CAD build for the part. Positions are in the model's coordinates, mm. Round coordinates to 2 decimals unless told otherwise and drop trailing zeros. Write each loop counter-clockwise with the first axis right and the second up, starting at its lowest first coordinate (ties: lowest second). Pieces come first, ordered by that corner, then holes. Notation, with made-up numbers: (57.5, 21) -> (74.5, 21) arc R34 ccw to (74.5, 56) -> close; hole circle Ø2 at (-29, 36.25). An arc over 180 degrees is marked (long way). Answer in a Markdown table with one row per item. Add a question column.
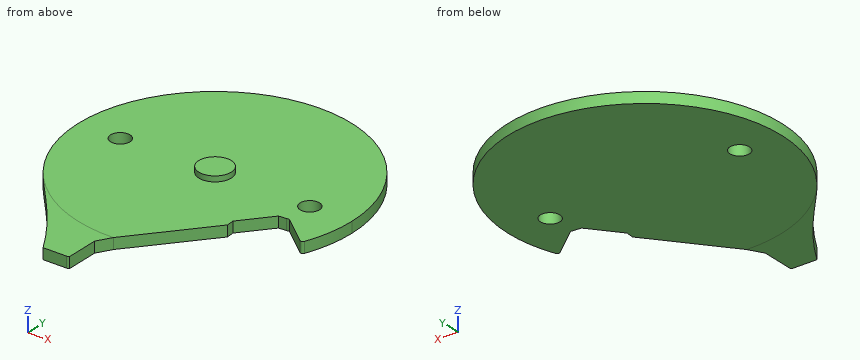
Autodesk Inventor part; units mm, degrees
ref_plane "YZ Plane" through (0, 0, 0) normal (1, 0, 0) x (0, 1, 0)
ref_plane "XZ Plane" through (0, 0, 0) normal (0, 1, 0) x (-1, 0, 0)
ref_plane "XY Plane" through (0, 0, 0) normal (0, 0, 1) x (1, 0, 0)
sketch "Skizze1" plane through (0, 0, 0) normal (0, 0, 1) x (1, 0, 0)
  circle A0 centre (0, 0) radius 12.625
  line L0 (31.2972, 39.0088) -> (31.2972, -40.1485) construction
  line L1 (31.2972, -40.1485) -> (-28.0708, -40.1485) construction
  line L2 (-28.0708, -40.1485) -> (-28.0708, 39.0088) construction
  line L3 (-28.0708, 39.0088) -> (31.2972, 39.0088) construction
  line L4 (-10.1529, -7.5039) -> (-9.5297, -8.4617) construction
  line L5 (-9.5297, -8.4617) -> (-6.7964, -11.288) construction
  line L6 (-6.7964, -11.288) -> (-4.1897, -14.7808) construction
  line L7 (-4.1897, -14.7808) -> (-3.5273, -15.9852) construction
  line L8 (-3.5273, -15.9852) -> (-2.9089, -17.0055) construction
  spline S0 degree 4 poles (-10.1529, -7.5039) (-10.1523, -7.5049) (-9.5297, -8.4617) (-6.7964, -11.288) (-4.1897, -14.7808) (-3.5273, -15.9852) (-2.9089, -17.0055) knots 1 1 1 1 1 2 3 4 4 4 4 4
  line L9 (-2.9089, -17.0055) -> (-0.7662, -17.0055)
  arc A1 (-0.7662, -17.0055) -> (-0.5189, -16.9237) centre (-0.7662, -16.5904) ccw
  line L10 (-0.5189, -16.9237) -> (-0.5189, -13.9001)
  line L11 (-0.5189, -13.9001) -> (0.2333, -12.6228)
  line L12 (0.2333, -12.6228) -> (8.5203, -2.5497)
  line L13 (8.809, -2.5289) -> (11.6496, -4.8659)
  line L14 (5.7065, -5.97) -> (5.6548, -5.2536)
  line L15 (5.6548, -5.2536) -> (7.8388, -2.5989)
  line L16 (7.8388, -2.5989) -> (8.809, -2.5289)
  dimension "d0" = 25.25
extrude "Extrusion1" add sketch "Skizze1" along normal blind 1 contours A0 L13 L16 L15 L14 L12 | A0 L11 L10 A1 L9 S0
fillet "Rundung1" radius 0.2 2 edges at (11.6496, -4.8659, 0.5) (8.5203, -2.5497, 0.5)
sketch "Skizze2" plane through (0, 0, 1) normal (0, 0, 1) x (1, 0, 0)
  circle A0 centre (0, 0) radius 1.5
  dimension "d46" = 3
extrude "Extrusion2" add sketch "Skizze2" along normal blind 0.5
sketch "Skizze3" plane through (0, 0, 1) normal (0, 0, 1) x (1, 0, 0)
  line L0 (-8.75, 0) -> (8.75, 0) construction
  circle A0 centre (-8.75, 0) radius 0.9
  circle A1 centre (8.75, 0) radius 0.9
  point P0 (0, 0)
  dimension "d49" = 17.5
  dimension "d50" = 8.75
  dimension "d51" = 1.8
  dimension "d52" = 1.8
extrude "Extrusion3" cut sketch "Skizze3" against normal through all
equation "\"d52\" = d51"
properties part number "pcb"
Item 1: Saw through at A-A on z = 0.6. Count the separate pieces of the cut face and the enclosed holes in it, then the cut area to 3 significant figures.
Item 2: Saw through at C-C on y = 7.75. Give the cut face in (x, z), then the cut area to 3 significant figures.
Item 3: Drill centre lines: probe 1 along Z at (x, y) = (0.5, 5.25); probe 2 along Y at (x, z) = (-8.75, 0.35); probe 3 along Y at (x, z) = (8.75, 0.65). Where is each one in solid material? Low to high.
Item 4: Pin check, flat tips, straight feed: pin 1 (0.8 mm diameter, centred on y = -15, z = 0.5, fed in from +X); pin 2 (1.1 mm diameter, centred on x = 8.75, y = 0, fed in from -Z); pin 3 (3 mm diameter, centred on x = -7, y = -12.5, fed in from +Z). Stop position of each tip, or through.
Item 5: Saw through at B-B on x = 10. Give the cut face in (y, z), then the cut area to 3 significant figures.
Recorded:
| question | item | result |
|---|---|---|
| 1 | separate pieces | 1 |
| 1 | enclosed holes | 2 |
| 1 | area | 471 mm2 |
| 2 | outline | (-9.97, 0) -> (9.97, 0) -> (9.97, 1) -> (-9.97, 1) -> close |
| 2 | area | 19.9 mm2 |
| 3 | probe 1 | 0 to 1 |
| 3 | probe 2 | -9.24 to -0.9, 0.9 to 9.1 |
| 3 | probe 3 | -2.53 to -0.9, 0.9 to 9.1 |
| 4 | pin 1 | x = -0.52 |
| 4 | pin 2 | through |
| 4 | pin 3 | z = 1 |
| 5 | outline | (-3.51, 0) -> (7.71, 0) -> (7.71, 1) -> (-3.51, 1) -> close |
| 5 | area | 11.2 mm2 |
